Autodesk Fusion 360 part; units mm, degrees
sketch "Sketch1" plane through (0, 0, 0) normal (0, 0, 1) x (1, 0, 0)
  line L0 (82.55, 24.892) -> (-82.55, 24.892)
  line L1 (-82.55, 24.892) -> (-82.55, -24.892)
  line L2 (-82.55, -24.892) -> (82.55, -24.892)
  line L3 (82.55, -24.892) -> (82.55, 24.892)
  line L4 (82.55, 24.892) -> (-82.55, -24.892) construction
  line L5 (-82.55, 24.892) -> (82.55, -24.892) construction
  circle A0 centre (-49.2125, -1.016) radius 3.9688
  circle A1 centre (49.2125, -1.016) radius 3.9688
  line L6 (-39.4335, -1.016) -> (-39.4335, -24.892)
  line L7 (-58.9915, -1.016) -> (-58.9915, -24.892)
  line L8 (39.4335, -1.016) -> (39.4335, -24.892)
  line L9 (58.9915, -1.016) -> (58.9915, -24.892)
  arc A2 (-39.4335, -1.016) -> (-58.9915, -1.016) centre (-49.2125, -1.016) ccw
  arc A3 (58.9915, -1.016) -> (39.4335, -1.016) centre (49.2125, -1.016) ccw
  line L10 (0, 24.892) -> (0, -24.892) construction
  circle A4 centre (-49.2125, -1.016) radius 6.604
  circle A5 centre (49.2125, -1.016) radius 6.604
  line L11 (-42.6085, -1.016) -> (-42.6085, -24.892)
  line L12 (-55.8165, -1.016) -> (-55.8165, -24.892)
  line L13 (42.6085, -1.016) -> (42.6085, -24.892)
  line L14 (55.8165, -1.016) -> (55.8165, -24.892)
  point P0 (-49.2125, -1.016)
  point P1 (49.2125, -1.016)
  dimension "d1" = 165.1
  dimension "d2" = 49.784
  dimension "d3" = 7.9375
  dimension "d4" = 7.9375
  dimension "d5" = 98.425
  dimension "d9" = 23.876
  dimension "d10" = 19.558
  dimension "d11" = 19.558
  dimension "d16" = 23.876
  dimension "d17" = 49.2125
  dimension "d19" = 13.208
  dimension "d20" = 13.208
extrude "Extrude1" add sketch "Sketch1" against normal blind 24.384
extrude "Extrude2" cut sketch "Sketch1" against normal blind 15.24 contours L2 L8 L9 A3 A5 L13 L14 | L2 L6 L7 A2 A4 L11 L12 | L2 A5 L13 L14 | L2 A4 L11 L12 | A5 | A4
extrude "Extrude3" add sketch "Sketch1" against normal blind 7.3025 contours L2 L8 L9 A3 A5 L13 L14 | L2 L6 L7 A2 A4 L11 L12
equation "d2 = 2 in - 0.04 in"
equation "d4 = d3"
equation "d11 = d10"
equation "d12 = -1 in + 0.04 in"
equation "d17 = ( 3.875 / 2 ) * 1 in"
equation "d20 = d19"
Read the model definition and answer for the solid it produces. Units are mm, in the model's axes. A direction names the side the tool comes from. Coordinates: 2 decimals unless noted, no trailing zeros. Write each loop counter-clockwise with the first axis right and the second up, starting at its lowest first coordinate (ties: lowest second). Pieces come first, ordered by that corner, then holes. Notation, with made-up numbers: (5.25, 14) -> (12.25, 14) arc R27 cw to (12.25, 46) -> close; hole circle Ø11 at (11, 31). An arc over 180 degrees is marked (long way). Return JSON: item names as keys, results as strings.
1. Find the intervals of material crossed by line 1 along X through (y, z) = (-15, -13.75); line 2 along X through (y, z) = (-2, -3.75); line 3 along Z through (x, y) = (54, -6), in increasing order. Write a range as from..to.
Found:
{"line 1": "-82.55..-58.99, -39.43..39.43, 58.99..82.55", "line 2": "-82.55..-55.82, -42.61..42.61, 55.82..82.55", "line 3": "-24.38..-15.24"}
2. A cutting plane is placed at B-B (z = -4.75). Determine the outline of the cut face in (x, y), and give its area (3 significant figures).
Found:
{"outline": "(-82.55, -24.89) -> (-55.82, -24.89) -> (-55.82, -1.02) arc R6.6 cw to (-42.61, -1.02) -> (-42.61, -24.89) -> (42.61, -24.89) -> (42.61, -1.02) arc R6.6 cw to (55.82, -1.02) -> (55.82, -24.89) -> (82.55, -24.89) -> (82.55, 24.89) -> (-82.55, 24.89) -> close", "area": "7,450 mm2"}
3. A cutting plane is placed at A-A (y = -3.5). Determine the outline of the cut face in (x, z).
Found:
{"outline": "(-82.55, -24.38) -> (-52.31, -24.38) -> (-52.31, -15.24) -> (-58.99, -15.24) -> (-58.99, -7.3) -> (-55.82, -7.3) -> (-55.82, 0) -> (-82.55, 0) -> close; (-46.12, -24.38) -> (46.12, -24.38) -> (46.12, -15.24) -> (39.43, -15.24) -> (39.43, -7.3) -> (42.61, -7.3) -> (42.61, 0) -> (-42.61, 0) -> (-42.61, -7.3) -> (-39.43, -7.3) -> (-39.43, -15.24) -> (-46.12, -15.24) -> close; (52.31, -24.38) -> (82.55, -24.38) -> (82.55, 0) -> (55.82, 0) -> (55.82, -7.3) -> (58.99, -7.3) -> (58.99, -15.24) -> (52.31, -15.24) -> close"}
4. A cutting plane is placed at C-C (y = -20). Determine the outline of the cut face in (x, z), and give its area (3 significant figures).
Found:
{"outline": "(-82.55, -24.38) -> (82.55, -24.38) -> (82.55, 0) -> (55.82, 0) -> (55.82, -7.3) -> (58.99, -7.3) -> (58.99, -15.24) -> (39.43, -15.24) -> (39.43, -7.3) -> (42.61, -7.3) -> (42.61, 0) -> (-42.61, 0) -> (-42.61, -7.3) -> (-39.43, -7.3) -> (-39.43, -15.24) -> (-58.99, -15.24) -> (-58.99, -7.3) -> (-55.82, -7.3) -> (-55.82, 0) -> (-82.55, 0) -> close", "area": "3,520 mm2"}
5. Determine the mould class of faces 1 (the face through (49.358, 5.586, -3.6)), 2 (the face through (39.434, -13, -11)) for opening direction Z: pulls with the +Z half, pulls with the -Z half, needs draft (parallel to the pull), parting line crosses it, or undercut.
Found:
{"face 1": "needs draft", "face 2": "undercut"}
6. A tool of negligible diameter and unlimited length cuts with its end or side. For faces 3 (the face through (-82.55, 0, -12)), 4 (the face through (-49, 8.76, -11.22)), 5 (the face through (-55.816, -13, -4)), from which of +Z, -Z, +X, -X, +Y, -Y can it reach the whole face along a straight path? Write none if from no direction.
Found:
{"face 3": "+Z, -Z, -X, +Y, -Y", "face 4": "-Y", "face 5": "+Z, -Y"}
